```python
from build123d import *

# Parameters (mm, degrees)
SKETCH1_R           = 13.97
SKETCH1_R_2         = 3.556
SKETCH1_R_3         = 1.5875
BOSS_EXTRUDE4_DEPTH = 2.54
SKETCH2_R           = 2.159
SKETCH2_R_2         = 1.5875
BOSS_EXTRUDE6_DEPTH = 3.048
BOSS_EXTRUDE7_START = 3.302
SKETCH3_R           = 13.97
SKETCH3_R_2         = 2.921
BOSS_EXTRUDE7_DEPTH = 3.302


with BuildPart() as part:
    # Sketch1 → Boss-Extrude4 (new body)
    with BuildSketch(Plane(origin=(0, 0, 0), x_dir=(1, 0, 0), z_dir=(0, 1, 0))):
        with Locations(Location((0, 0, 0), (0, 0, 270))):
            Circle(SKETCH1_R)
        with Locations(Location((0, 0, 0), (0, 0, 270))):
            Circle(SKETCH1_R_2, mode=Mode.SUBTRACT)
        with Locations(Location((-7.9502, 0, 0), (0, 0, 270))):
            Circle(SKETCH1_R_3, mode=Mode.SUBTRACT)
        with Locations(Location((7.9502, 0, 0), (0, 0, 270))):
            Circle(SKETCH1_R_3, mode=Mode.SUBTRACT)
        with Locations(Location((0, 9.271, 0), (0, 0, 270))):
            Circle(SKETCH1_R_3, mode=Mode.SUBTRACT)
        with Locations(Location((0, -9.271, 0), (0, 0, 270))):
            Circle(SKETCH1_R_3, mode=Mode.SUBTRACT)
    extrude(amount=BOSS_EXTRUDE4_DEPTH)

    # Sketch2 → Boss-Extrude6 (add)
    # profile 1 of 4: a face of its own
    with BuildSketch(Plane(origin=(0, 2.54, 0), x_dir=(1, 0, 0), z_dir=(0, 1, 0))):
        with Locations(Location((0, 9.271, 0), (0, 0, 90))):
            Circle(SKETCH2_R)
        with Locations(Location((0, 9.271, 0), (0, 0, 270))):
            Circle(SKETCH2_R_2, mode=Mode.SUBTRACT)
    # profile 2 of 4: a face of its own
    with BuildSketch(Plane(origin=(0, 2.54, 0), x_dir=(1, 0, 0), z_dir=(0, 1, 0))):
        with Locations(Location((7.9502, 0, 0), (0, 0, 90))):
            Circle(SKETCH2_R)
        with Locations(Location((7.9502, 0, 0), (0, 0, 270))):
            Circle(SKETCH2_R_2, mode=Mode.SUBTRACT)
    # profile 3 of 4: a face of its own
    with BuildSketch(Plane(origin=(0, 2.54, 0), x_dir=(1, 0, 0), z_dir=(0, 1, 0))):
        with Locations(Location((-7.9502, 0, 0), (0, 0, 90))):
            Circle(SKETCH2_R)
        with Locations(Location((-7.9502, 0, 0), (0, 0, 270))):
            Circle(SKETCH2_R_2, mode=Mode.SUBTRACT)
    # profile 4 of 4: a face of its own
    with BuildSketch(Plane(origin=(0, 2.54, 0), x_dir=(1, 0, 0), z_dir=(0, 1, 0))):
        with Locations(Location((0, -9.271, 0), (0, 0, 90))):
            Circle(SKETCH2_R)
        with Locations(Location((0, -9.271, 0), (0, 0, 270))):
            Circle(SKETCH2_R_2, mode=Mode.SUBTRACT)
    extrude(amount=BOSS_EXTRUDE6_DEPTH)

    # Sketch3 → Boss-Extrude7 (add)
    with BuildSketch(Plane(origin=(0, 0, 0), x_dir=(-1, 0, 0), z_dir=(0, -1, 0)).offset(BOSS_EXTRUDE7_START)):
        with Locations(Location((0, 0, 0), (0, 0, 90))):
            Circle(SKETCH3_R)
        with Locations(Location((0, -9.271, 0), (0, 0, 270))):
            Circle(SKETCH3_R_2, mode=Mode.SUBTRACT)
        with Locations(Location((-7.9502, 0, 0), (0, 0, 270))):
            Circle(SKETCH3_R_2, mode=Mode.SUBTRACT)
        with BuildLine():
            ThreePointArc((-3.556, 0), (-2.514471714, 2.514471714), (0, 3.556))
            ThreePointArc((0, 3.556), (2.514471714, 2.514471714), (3.556, 0))
            ThreePointArc((3.556, 0), (0, -3.556), (-3.556, 0))
        make_face(mode=Mode.SUBTRACT)
        with Locations(Location((7.9502, 0, 0), (0, 0, 270))):
            Circle(SKETCH3_R_2, mode=Mode.SUBTRACT)
        with BuildLine():
            ThreePointArc((2.921, 9.271), (2.065458908, 7.205541092), (0, 6.35))
            ThreePointArc((0, 6.35), (-2.065458908, 11.336458908), (2.921, 9.271))
        make_face(mode=Mode.SUBTRACT)
    extrude(amount=-BOSS_EXTRUDE7_DEPTH)


solid = part.part
```
Check sheet for the modelled part. Datum: model origin and axes. Units: mm. A direction names the side the tool comes from. Round coordinates to 2 decimals unless told otherwise and drop trailing zeros. Order: outer loops, then holes, each group sorted by start corner. A loop starts at its lowest first (then second) coordinate and runs counter-clockwise, first axis right, second up. Notation, with made-up numbers: (32, 50) - (59, 50) arc R11 cw to (59, 59) - close; hole circle Ø1 at (3.25, -30). An arc over 180 degrees is marked (long way). Answer as CSV lines item,"result". Start each with the question number.
1) Depth check by flat-ended pin: pin 1 (4 mm diameter, centred on x = -7.95, z = 0, fed in from -Y); pin 2 (8 mm diameter, centred on x = 7, z = -9, fed in from +Y); pin 3 (3 mm diameter, centred on y = -1, z = -5, fed in from +X). Enter the tip coordinate at first touch or a pass-through.
2) Scan lines: probe 1 along X at (y, z) = (2.7, 0); probe 2 along X at (y, z) = (4.25, 9.25); probe 3 along X at (y, z) = (2, 0.25). Record each from-to range of solid material in increasing order.
3) Section check A-A (y = 5). Record the cut outline in (x, z) (1 decimal).
4) Draft check along X on faces 4 (the face through (-1.3, 0, -8)), 5 (the face through (-2.14, 4.04, -8.99)), 6 (the face through (6, 5.588, 0)). Enter one of: +X half, -X half, draft (parallel to the pull), parting line (faces both ways), or undercut.
5) Section check B-B (x = -2.5). Record the cut outline in (y, z).
6) Section check C-C (y = 0.5). Record the cut outline in (x, z) (1 decimal).
7) Section check D-D (y = -1.75). Record the cut outline in (x, z).
8) Tool access check on faces 1 (the face through (-1, 5.588, 11)), 2 (the face through (-1, 0, 11)), 3 (the face through (9.264, 4.043, 1.713)). Record the directions out of +Z, -Z, +X, -X, +Y, -Y that give a thin tool (end or side, any length) a straight path to the whole face; none if there is none.
Determined:
1,pin 1,"y = 0"
1,pin 2,"y = 2.54"
1,pin 3,"x = 13.52"
2,probe 1,"-10.11 to -9.54, -6.36 to -5.79, 5.79 to 6.36, 9.54 to 10.11"
2,probe 2,"-2.16 to -1.59, 1.59 to 2.16"
2,probe 3,"-13.97 to -9.52, -6.38 to -3.55, 3.55 to 6.38, 9.52 to 13.97"
3,outline,"circle Ø4.3 at (-8, 0); circle Ø4.3 at (0, -9.3); circle Ø4.3 at (0, 9.3); circle Ø4.3 at (8, 0); hole circle Ø3.2 at (-8, 0); hole circle Ø3.2 at (0, -9.3); hole circle Ø3.2 at (0, 9.3); hole circle Ø3.2 at (8, 0)"
4,face 4,"undercut"
4,face 5,"parting line"
4,face 6,"draft"
5,outline,"(-3.3, -13.74) - (2.54, -13.74) - (2.54, -2.53) - (-3.3, -2.53) - (-3.3, -7.76) - (0, -7.76) - (0, -10.78) - (-3.3, -10.78) - close; (-3.3, 2.53) - (2.54, 2.53) - (2.54, 13.74) - (-3.3, 13.74) - (-3.3, 10.78) - (0, 10.78) - (0, 7.76) - (-3.3, 7.76) - close"
6,outline,"circle Ø27.9 at (0, 0); hole circle Ø3.2 at (-8, 0); hole circle Ø7.1 at (0, 0); hole circle Ø3.2 at (0, -9.3); hole circle Ø3.2 at (0, 9.3); hole circle Ø3.2 at (8, 0)"
7,outline,"circle Ø27.94 at (0, 0); hole circle Ø5.84 at (-7.95, 0); hole circle Ø7.11 at (0, 0); hole circle Ø5.84 at (0, -9.27); hole circle Ø5.84 at (0, 9.27); hole circle Ø5.84 at (7.95, 0)"
8,face 1,"+Z, -Z, +X, -X, +Y"
8,face 2,"-Y"
8,face 3,"+Y"
